```python
from build123d import *

# Parameters (mm, degrees)
SKETCH1_W                                        = 100
SKETCH1_H                                        = 55
BOSS_EXTRUDE1_DEPTH                              = 5
CBORE_FOR_M3_PAN_HEAD_MACHINE_SCREW1_D           = 3.6
CBORE_FOR_M3_PAN_HEAD_MACHINE_SCREW1_CBORE_D     = 7
CBORE_FOR_M3_PAN_HEAD_MACHINE_SCREW1_CBORE_DEPTH = 2.4
MIRROR1_AT_THE_SECOND_PLANE_COPY_1_D             = 3.6
MIRROR1_AT_THE_SECOND_PLANE_COPY_1_CBORE_D       = 7
MIRROR1_AT_THE_SECOND_PLANE_COPY_1_CBORE_DEPTH   = 2.4
BOSS_EXTRUDE3_DEPTH                              = 15
BOSS_EXTRUDE3_DEPTH_BACK                         = 5
SKETCH11_W                                       = 100
SKETCH11_H                                       = 11.02
SKETCH11_H_2                                     = 5
BOSS_EXTRUDE5_DEPTH                              = 5


with BuildPart() as part:
    # Sketch1 → Boss-Extrude1 (new body)
    with BuildSketch(Plane(origin=(0, 0, 0), x_dir=(1, 0, 0), z_dir=(0, 1, 0))):
        with Locations((50, -27.5)):
            Rectangle(SKETCH1_W, SKETCH1_H)
    extrude(amount=BOSS_EXTRUDE1_DEPTH)

    # CBORE for M3 Pan Head Machine Screw1 (through all)
    with Locations(Plane(origin=(0, 0, 0), x_dir=(-1, 0, 0), z_dir=(0, -1, 0))):
        with Locations((-10, -12.5)):
            cbore_for_m3_pan_head_machine_screw1 = CounterBoreHole(CBORE_FOR_M3_PAN_HEAD_MACHINE_SCREW1_D / 2, CBORE_FOR_M3_PAN_HEAD_MACHINE_SCREW1_CBORE_D / 2, CBORE_FOR_M3_PAN_HEAD_MACHINE_SCREW1_CBORE_DEPTH)

    # Mirror1: CBORE for M3 Pan Head Machine Screw1 across plane
    add(cbore_for_m3_pan_head_machine_screw1.mirror(Plane.XY.offset(27.5)), mode=Mode.SUBTRACT)

    # Mirror1 at the second plane: CBORE for M3 Pan Head Machine Screw1 across plane
    add(cbore_for_m3_pan_head_machine_screw1.mirror(Plane.ZY.offset(-25)), mode=Mode.SUBTRACT)

    # Mirror1 at the second plane copy 1 (through all)
    with Locations(Plane(origin=(50, 0, 55), x_dir=(1, 0, 0), z_dir=(0, -1, 0))):
        with Locations((-10, -12.5)):
            CounterBoreHole(MIRROR1_AT_THE_SECOND_PLANE_COPY_1_D / 2, MIRROR1_AT_THE_SECOND_PLANE_COPY_1_CBORE_D / 2, MIRROR1_AT_THE_SECOND_PLANE_COPY_1_CBORE_DEPTH)

    # Sketch9 → Boss-Extrude3 (add, two sides: drawn at the far end of the back side and taken through both)
    with BuildSketch(Plane(origin=(0, 5, 0), x_dir=(1, 0, 0), z_dir=(0, 1, 0)).offset(-BOSS_EXTRUDE3_DEPTH_BACK)):
        Polygon((-200, 0), (50, 0), (100, 0), (100, 30), (-200, 30), align=None)
    extrude(amount=BOSS_EXTRUDE3_DEPTH + BOSS_EXTRUDE3_DEPTH_BACK)

    # Sketch11 → Boss-Extrude5 (add)
    with BuildSketch(Plane(origin=(0, 20, 0), x_dir=(1, 0, 0), z_dir=(0, 1, 0))):
        with Locations((50, 24.49)):
            Rectangle(SKETCH11_W, SKETCH11_H)
        with Locations((50, 6.48)):
            Rectangle(SKETCH11_W, SKETCH11_H_2)
    extrude(amount=BOSS_EXTRUDE5_DEPTH)


solid = part.part
```
Input: part model. Units: mm. Frame: model coordinates. A direction names the side the tool comes from. Round coordinates to 2 decimals unless told otherwise and drop trailing zeros. Loops run counter-clockwise (first coordinate to the right, second up) from the corner with the lowest first, then second, coordinate; pieces in that order, holes last. Notation, with made-up numbers: (36, 63) -> (92, 63) arc R34 ccw to (92, 100) -> close; hole circle Ø2 at (-36, 12). An arc over 180 degrees is marked (long way). Write each question's results on one line, items separated by ' | '.
1. Ray query, line 1 (X direction, y = 3, z = 12.5); line 2 (Z direction, x = 10, y = 3.3); line 3 (Z direction, x = 40, y = 1.95). Return the intervals inside material, ascending. Write a range as from..to.
Geometry results:
line 1: 0..8.2, 11.8..38.2, 41.8..100 | line 2: -30..10.7, 14.3..40.7, 44.3..55 | line 3: -30..9, 16..39, 46..55
2. First-contact query: P1, Ø10, axis at x = -18.5, y = 14.5, coming from the +Z side; P2, Ø3.5, axis at x = 9.5, z = 13.5, coming from the -Y side; P3, Ø11, axis at x = 10, z = 12.5, coming from the +Y side. Flat tips, straight axial feed; report the tip coordinate or a pass-through.
Geometry results:
P1: z = 0 | P2: y = 2.4 | P3: y = 5
3. Section B-B (y = 15.75). Return loops of the section in (x, z).
Geometry results:
outline: (-200, -30) -> (100, -30) -> (100, 0) -> (-200, 0) -> close
4. Set-up query: faces 1 (the face through (49, 22, -8.98)), 2 (the face through (40, 1, 46)), 3 (the face through (49, 22, -3.98)). Return all of +Z, -Z, +X, -X, +Y, -Y with unobstructed straight access to the full face (end or side cutting, diameter ignored); none if empty.
Geometry results:
face 1: +X, -X, +Y | face 2: -Y | face 3: +Z, +X, -X, +Y
5. Mould query, pull axis Z, two halves, no side actions, for faces 4 (the face through (38, 2.4, 43)), 5 (the face through (-52, 10, -30)), 6 (the face through (0, 22, -24)), 7 (the face through (12, 2.4, 43)). Classes: +Z half, -Z half, draft (parallel to the pull), parting line (faces both ways), or undercut.
Geometry results:
face 4: undercut | face 5: -Z half | face 6: draft | face 7: undercut
6. Section A-A (x = 56.5). Return loops of the section in (y, z).
Geometry results:
outline: (0, -30) -> (25, -30) -> (25, -18.98) -> (20, -18.98) -> (20, -8.98) -> (25, -8.98) -> (25, -3.98) -> (20, -3.98) -> (20, 0) -> (5, 0) -> (5, 55) -> (0, 55) -> close
7. Section C-C (z = 29). Return loops of the section in (x, y).
Geometry results:
outline: (0, 0) -> (100, 0) -> (100, 5) -> (0, 5) -> close
